```python
from build123d import *

# Parameters (mm, degrees)
F1_DEPTH  = 12
F3_DEPTH  = 50
F4_R      = 3.15
F5_DEPTH  = 80.6785650794
F8_DEPTH  = 74.6785650794
F9_R      = 3.15
F10_DEPTH = 57.126
F12_DEPTH = 3


with BuildPart() as f1:
    # F0 (on Top) → F1 (new body)
    with BuildSketch(Plane.XY):
        with BuildLine():
            ThreePointArc((36.8699149036, -7.5), (-37.625, 0), (36.8699149036, 7.5))
            Line((36.8699149036, 7.5), (53.6314719497, 7.5))
            Line((53.6314719497, 7.5), (53.6314719497, 15.5))
            Line((53.6314719497, 15.5), (38.6314719497, 15.5))
            ThreePointArc((38.6314719497, 15.5), (22.0370581838, 35.3130102314), (-3.0526031231, 41.5129165342))
            ThreePointArc((-3.0526031231, 41.5129165342), (-41.625, 0), (-3.0526031231, -41.5129165342))
            ThreePointArc((-3.0526031231, -41.5129165342), (22.0370581838, -35.3130102314), (38.6314719497, -15.5))
            Line((38.6314719497, -15.5), (53.6314719497, -15.5))
            Line((53.6314719497, -15.5), (53.6314719497, -7.5))
            Line((53.6314719497, -7.5), (36.8699149036, -7.5))
        make_face()
        with BuildLine():
            ThreePointArc((-3.0526031231, -41.5129165342), (-41.625, 0), (-3.0526031231, 41.5129165342))
            Line((-3.0526031231, 41.5129165342), (-57.625, 37.5))
            Line((-57.625, 37.5), (-57.625, -37.5))
            Line((-57.625, -37.5), (-3.0526031231, -41.5129165342))
        make_face()
    extrude(amount=F1_DEPTH)

    # F2 (on Front) → F3 (cut, symmetric)
    with BuildSketch(Plane.XZ):
        Polygon((-57.6562229203, 26.0493437853), (-57.6562229203, 2.8076118446), (-48.4638347648, 12), (-48.4638347648, 26.0493437853), align=None)
    extrude(amount=F3_DEPTH, both=True, mode=Mode.SUBTRACT)

    # F4 (on face) → F5 (cut, through all)
    with BuildSketch(Plane(origin=(-30.2319173824, 0, 30.2319173824), x_dir=(0.7071067812, 0, 0.7071067812), z_dir=(-0.7071067812, 0, 0.7071067812))):
        with Locations((-32.2617468916, 30)):
            Circle(F4_R)
        with Locations((-32.2617468916, -30)):
            Circle(F4_R)
    extrude(amount=-F5_DEPTH, mode=Mode.SUBTRACT)

    # F7 (on offset) → F8 (cut, through all)
    with BuildSketch(Plane(origin=(-25.9892766953, 0, 25.9892766953), x_dir=(0.7071067812, 0, 0.7071067812), z_dir=(-0.7071067812, 0, 0.7071067812))):
        Polygon((-32.2617468916, 24.1110272543), (-27.1617468916, 27.0555136271), (-27.1617468916, 32.9444863729), (-32.2617468916, 35.8889727457), (-37.3617468916, 32.9444863729), (-37.3617468916, 27.0555136271), align=None)
        Polygon((-32.2617468916, -35.8889727457), (-27.1617468916, -32.9444863729), (-27.1617468916, -27.0555136271), (-32.2617468916, -24.1110272543), (-37.3617468916, -27.0555136271), (-37.3617468916, -32.9444863729), align=None)
    extrude(amount=-F8_DEPTH, mode=Mode.SUBTRACT)

    # F9 (on face) → F10 (cut, through all)
    with BuildSketch(Plane.XZ.offset(15.5)):
        with Locations((46.1314719497, 6)):
            Circle(F9_R)
    extrude(amount=-F10_DEPTH, mode=Mode.SUBTRACT)

    # F11 (on face) → F12 (cut)
    with BuildSketch(Plane.XZ.offset(15.5)):
        Polygon((49.0759583226, 0.9), (52.0204446954, 6), (49.0759583226, 11.1), (43.1869855768, 11.1), (40.242499204, 6), (43.1869855768, 0.9), align=None)
    extrude(amount=-F12_DEPTH, mode=Mode.SUBTRACT)


solid = f1.part
```
Input: part model. Units: mm. Frame: model coordinates. A direction names the side the tool comes from. Give positions to 0.01 mm unless a question says otherwise; leave off trailing zeros. Write each loop counter-clockwise with the first axis right and the second up, starting at its lowest first coordinate (ties: lowest second). Pieces come first, ordered by that corner, then holes. Notation, with made-up numbers: (55, 44) - (107, 44) arc R20 cw to (107, 83) - close; hole circle Ø1 at (59, 80.25). An arc over 180 degrees is marked (long way). Write item = value, one per line. Start each with the question number.
1) Cut plane C-C (x = 47.5). Return loops of the section in (y, z).
2) Draft query along X for faces 4 (the face through (43, 7.5, 3)), 5 (the face through (-29.957, 39.535, 5.916)), 6 (the face through (-49.92, -32.79, 6.36)). Return one class per face: pulls with the +X half, pulls with the -X half, needs draft (parallel to the pull), parting line crosses it, or undercut.
3) Pin query (flat end, axial travel): pin 1 (5 mm diameter, centred on x = 33.5, z = 2.5, fed in from -Y); pin 2 (3 mm diameter, centred on x = -44.5, z = 10.5, fed in from +Y); pin 3 (5 mm diameter, centred on x = 24, y = 23, fed in from -Z); pin 4 (4 mm diameter, centred on y = -1.5, z = 6.5, fed in from -X). Return the tip coordinate at first contact, or that it passes through.
4) Cut plane A-A (x = 33.5). Return loops of the section in (y, z).
5) Cut plane D-D (x = 0). Return loops of the section in (y, z) (3 decimals).
6) Material intervals for L1, parallel to Y at x = 0, z = 3.75 (3 decimals); L2, parallel to Y at x = 3, z = 6.25; L3, parallel to X at y = 16.5, z = 2 (3 decimals), sorted ascending. Write a range as [from, to].
7) Reachability of faces 1 (the face through (-46.37, 30.08, 5.61)), 2 (the face through (-30.72, -39.48, 5.92)), 3 (the face through (41.69, -14.02, 3.49)) from +Z, -Z, +X, -X, +Y, -Y: full face, straight path, thin tool, end or side. Return the list, or none.
8) Cut plane B-B (y = 0). Return loops of the section in (x, z) (3 decimals), and give its area (3 significant figures).
Answers follow:
q1.outline = (-15.5, 0) - (-7.5, 0) - (-7.5, 3.16) - (-12.5, 3.16) - (-12.5, 0.9) - (-15.5, 0.9) - close; (-15.5, 11.1) - (-12.5, 11.1) - (-12.5, 8.84) - (-7.5, 8.84) - (-7.5, 12) - (-15.5, 12) - close; (7.5, 0) - (15.5, 0) - (15.5, 3.16) - (7.5, 3.16) - close; (7.5, 8.84) - (15.5, 8.84) - (15.5, 12) - (7.5, 12) - close
q2.face_4 = needs draft
q2.face_5 = pulls with the -X half
q2.face_6 = undercut
q3.pin_1 = -27.78
q3.pin_2 = 38.58
q3.pin_3 = through
q3.pin_4 = -55.96
q4.outline = (-24.71, 0) - (-17.13, 0) - (-17.13, 12) - (-24.71, 12) - close; (17.13, 0) - (24.71, 0) - (24.71, 12) - (17.13, 12) - close
q5.outline = (-41.625, 0) - (-37.625, 0) - (-37.625, 12) - (-41.625, 12) - close; (37.625, 0) - (41.625, 0) - (41.625, 12) - (37.625, 12) - close
q6.L1 = [-41.625, -37.625], [37.625, 41.625]
q6.L2 = [-41.52, -37.51], [37.51, 41.52]
q6.L3 = [-57.625, -33.814], [33.814, 38.215]
q7.face_1 = none
q7.face_2 = +Z, -Z, -X, -Y
q7.face_3 = -Y
q8.outline = (-57.625, 0) - (-37.625, 0) - (-37.625, 12) - (-48.464, 12) - (-57.625, 2.839) - close
q8.area = 198 mm^2
